Autodesk Inventor part; units mm, degrees
ref_plane "YZ Plane" through (0, 0, 0) normal (1, 0, 0) x (0, 1, 0)
ref_plane "XZ Plane" through (0, 0, 0) normal (0, 1, 0) x (-1, 0, 0)
ref_plane "XY Plane" through (0, 0, 0) normal (0, 0, 1) x (1, 0, 0)
sketch "Sketch2" plane through (0, 0, 0) normal (0, 0, 1) x (1, 0, 0)
  line L0 (-31.2032, 0) -> (39.8239, 0) construction
  line L1 (20.125, 19.3) -> (20.125, 21.675)
  line L2 (20.125, 21.675) -> (-20.125, 22.85)
  line L3 (-20.125, 22.85) -> (-20.125, 19.3)
  line L4 (0, 19.3) -> (0, 0) construction
  line L5 (8.775, 19.3) -> (8.775, 18.8)
  line L6 (8.775, 18.8) -> (9.475, 18.8)
  line L7 (9.475, 18.8) -> (9.475, 19.3)
  line L8 (-20.125, 19.3) -> (8.775, 19.3)
  line L9 (9.475, 19.3) -> (20.125, 19.3)
  line L10 (0, 22.2625) -> (0, 19.3) construction
  dimension "d2" = 40.25
  dimension "d34" = 0.5
  dimension "d36" = 0.7
  dimension "d41" = 19.3
  dimension "d45" = 11.35
  dimension "d46" = 22.85
  dimension "d47" = 21.675
revolve "Revolution1" add sketch "Sketch2" angle 270 about axis through (-31.2032, 0, 0) along (1, 0, 0)
sketch "Sketch3" plane through (0, 0, 0) normal (0, 1, 0) x (-1, 0, 0)
  line L0 (20.125, 0) -> (20.125, -22.85)
  line L1 (20.125, -22.85) -> (20.125, -22.85)
  line L2 (20.125, -22.85) -> (20.125, 0)
  line L3 (20.125, 0) -> (20.125, 0)
  line L4 (-20.125, -19.3) -> (-20.125, -21.675)
  line L5 (-20.125, -21.675) -> (-20.125, 0)
  line L6 (-2.725, -5) -> (-2.725, 0)
  line L7 (9.125, -5) -> (-2.725, -5)
  line L8 (-20.125, -21.675) -> (20.125, -22.85)
  line L9 (20.125, -22.85) -> (-20.125, -21.675)
  line L10 (-2.725, 0) -> (-20.125, 0)
  line L11 (20.125, 0) -> (9.125, 0)
  line L12 (9.125, 0) -> (9.125, -5)
  dimension "d21" = 11
  dimension "d23" = 5
  dimension "d43" = 11.85
extrude "Extrusion1" cut sketch "Sketch3" against normal blind 200
sketch "Sketch4" plane through (0, 0, 0) normal (0, 1, 0) x (-1, 0, 0)
  line L0 (-20.125, 0) -> (20.125, 0)
  line L1 (9.125, 0) -> (-2.725, 0)
  line L2 (-2.725, 0) -> (-2.725, 6)
  line L3 (-2.725, 6) -> (9.125, 6)
  line L4 (9.125, 6) -> (9.125, 0)
  line L5 (20.125, 22.85) -> (20.125, 0)
  line L6 (-20.125, 21.675) -> (-20.125, 0)
  point P0 (-2.725, 0)
  dimension "d24" = 6
  dimension "d25" = 11
  dimension "d44" = 11.85
extrude "Extrusion2" cut sketch "Sketch4" along normal blind 200
chamfer "Chamfer1" distance 1.5 angle 45 1 edges at (20.125, 0, 21.675)
properties part number "PLASTIC_PART"
Model file for the job. Use its own axes, mm. A direction names the side the tool comes from. Give positions to 0.01 mm unless a question says otherwise; leave off trailing zeros. Write each loop counter-clockwise with the first axis right and the second up, starting at its lowest first coordinate (ties: lowest second). Pieces come first, ordered by that corner, then holes. Notation, with made-up numbers: M 52,72.25 L 78,72.25 A16 ccw 78,103.25 Z; hole C 74.5,8.5 d3. An arc over 180 degrees is marked long. One line per item, written item: value. Start each with the question number.
Q1. 3-axis set-ups, long thin cutter, end or side, ignore diameter. For faces 1 (the flat face through (11, -20, 0)), 2 (the flat face through (-9.125, -21, -2)), 3 (the flat face through (8.775, 0, 19)), 4 (the cylindrical face through (14.875, 0.424, 19.295)), 5 (the flat face through (2.725, 20, 3)): which of +Z, -Z, +X, -X, +Y, -Y reach the whole face in a straight line?
Q2. Saw through at A-A, the plane y = 0. Write the cut outline in (x, z) (3 decimals).
Q3. Saw through at B-B, the plane z = 1. State how many separate pieces and enclosed holes the cut face has, plus the area to 3 significant figures.
Q4. Probe probe 1 along X at (y, z) = (19, 5.5) (3 decimals); probe 2 along Z at (x, y) = (-1.5, 5); probe 3 along Y at (x, z) = (8.5, 9). List the from-to ranges inside material, lowest first. Write a range as [from, to].
Q5. Two-plate mould, pull along Y, no slides. Class faces 6 (the conical face through (-1.021, -3.05, 22.083)), 7 (the flat face through (2.725, -20, -3)), 8 (the cylindrical face through (9.13, 0.413, 18.795)): +Y half, -Y half, draft (parallel to the pull), parting line (faces both ways), or undercut.
Q6. Drop flat-ended pins along their axis: pin 1 Ø2 at (y, z) = (17.5, 5) entering from +X (3 decimals); pin 2 Ø2.5 at (x, y) = (15.5, -20) entering from -Z; pin 3 Ø3 at (y, z) = (-19.5, -3) entering from -X (3 decimals); pin 4 Ø9.5 at (y, z) = (8, 7.5) entering from -X. Give the stop position or say it passes through.
Q7. Saw through at C-C, the plane x = -10. Write the cut outline in (y, z), plus the area to 3 significant figures.
Output values:
1. face 1: -Z, +X, +Y, -Y
1. face 2: -Z, -X, +Y, -Y
1. face 3: -Z, -X
1. face 4: -Z, +X
1. face 5: -Z, +Y
2. outline: M -20.125,19.3 L 8.775,19.3 L 8.775,18.8 L 9.475,18.8 L 9.475,19.3 L 20.125,19.3 L 20.125,20.175 L 18.626,21.719 L -20.125,22.85 Z
3. separate pieces: 3
3. enclosed holes: 0
3. area: 201 mm²
4. probe 1: x = [-20.125, -9.125], [2.725, 20.125]
4. probe 2: z = [18.64, 21.74]
4. probe 3: y = [-20.09, -17.07], [17.07, 20.09]
5. face 6: parting line
5. face 7: draft
5. face 8: undercut
6. pin 1: stops at x = 9.475
6. pin 2: stops at z = 0
6. pin 3: stops at x = -9.125
6. pin 4: passes through
7. outline: M -22.55,0 L -19.3,0 A19.3 cw 19.3,0 L 22.55,0 A22.55 ccw Z
7. area: 214 mm²
